Check sheet for the modelled part. Datum: model origin and axes. Units: mm. A direction names the side the tool comes from. Round coordinates to 2 decimals unless told otherwise and drop trailing zeros. Order: outer loops, then holes, each group sorted by start corner. A loop starts at its lowest first (then second) coordinate and runs counter-clockwise, first axis right, second up. Notation, with made-up numbers: M 69.5,9 L 84.5,9 A31 ccw 84.5,34 Z; hole C 56,-36.5 d7. An arc over 180 degrees is marked long. One line per item, written item: value. Start each with the question number.
(1) Access from +Z, -Z, +X, -X, +Y, -Y to the whole of each face (thin tool, end or side, straight path). Record for faces 4 (the face through (9, 1, 129)), 5 (the face through (90.51, 1.23, 121.35)).
(2) Cross-section at B-B, the plane x = 37.5. Enter the section's corners in (y, z), and give its area (3 significant figures).
(3) Thickness scan on L1, parallel to Z at x = 41, y = 1.75; L2, parallel to Z at x = 57, y = 1; L3, parallel to Z at x = 66, y = 1.3. Record the ranges inside material, lowest first.
(4) Cross-section at D-D, the plane x = 69. Enter the section's corners in (y, z), and give its area (3 significant figures).
(5) Cross-section at C-C, the plane z = 41. Enter the section's corners in (x, y), and give its area (3 significant figures).
(6) Cross-section at A-A, the plane z = 66. Enter the section's corners in (x, y), and give its area (3 significant figures).
(7) Release check for a two-part mould opening along Z. For faces 1 (the face through (15.65, 1.23, 121.51)), 2 (the face through (49, 0, 62)), 3 (the face through (97, 1, 8)) record: released by +Z, released by -Z, zero draft, split by the parting line, or undercut.
(8) Depth check by flat-ended pin: pin 1 Ø1 at (y, z) = (1, 75) entering from +X; pin 2 Ø0.8 at (x, y) = (72, 0.5) entering from -Z; pin 3 Ø1.1 at (x, z) = (-4.5, 112.5) entering from +Y; pin 4 Ø1.2 at (x, y) = (72.5, 1) entering from +Z. Enter the tip coordinate at first touch or a pass-through.
from build123d import *

# Parameters (mm, degrees)
SKETCH1_W               = 106
SKETCH1_H               = 137
BOSS_EXTRUDE1_DEPTH     = 2.5
CUT_EXTRUDE1_DEPTH      = 174.237553665
CUT_EXTRUDE1_DEPTH_BACK = 174.237553665
SKETCH5_W               = 8
SKETCH5_H               = 8
SKETCH5_R               = 0.9
SKETCH5_W_2             = 9
BOSS_EXTRUDE4_DEPTH     = 2.5
CUT_EXTRUDE4_DEPTH      = 181.818278943
CUT_EXTRUDE4_DEPTH_BACK = 181.818278943
SKETCH3_R               = 1.2
SKETCH3_W               = 6.263237977
SKETCH3_H               = 0.25
SKETCH3_W_2             = 4.268245837
CUT_EXTRUDE5_DEPTH      = 181.818278943
CUT_EXTRUDE5_DEPTH_BACK = 181.818278943
SKETCH7_W               = 30
SKETCH7_H               = 12


with BuildPart() as part:
    # Sketch1 → Boss-Extrude1 (new body)
    with BuildSketch(Plane(origin=(0, 0, 0), x_dir=(1, 0, 0), z_dir=(0, 1, 0))):
        with Locations((53, -68.5)):
            Rectangle(SKETCH1_W, SKETCH1_H)
    extrude(amount=BOSS_EXTRUDE1_DEPTH)

    # Sketch2 → Cut-Extrude1 (cut, two sides: drawn at the far end of the back side and taken through both)
    with BuildSketch(Plane(origin=(0, 2.5, 0), x_dir=(1, 0, 0), z_dir=(0, 1, 0)).offset(-CUT_EXTRUDE1_DEPTH_BACK)):
        Polygon((60.5, -83.5), (96, -83.5), (96, -115.857864376), (84.857864376, -127), (60.5, -127), align=None)
        Polygon((106, -120), (89, -137), (106, -137), align=None)
        Polygon((17, -137), (0, -120), (0, -137), align=None)
        Polygon((45.5, -127), (21.142135624, -127), (10, -115.857864376), (10, -83.5), (45.5, -83.5), align=None)
        Polygon((10, -53.5), (45.5, -53.5), (45.5, -8), (23.142135624, -8), (10, -21.142135624), align=None)
        Polygon((60.5, -53.5), (60.5, -8), (82.857864376, -8), (96, -21.142135624), (96, -53.5), align=None)
        Polygon((106, 0), (89, 0), (106, -17), align=None)
        Polygon((0, 0), (0, -17), (17, 0), align=None)
    extrude(amount=CUT_EXTRUDE1_DEPTH + CUT_EXTRUDE1_DEPTH_BACK, mode=Mode.SUBTRACT)

    # Sketch5 → Boss-Extrude4 (add)
    # profile 1 of 8: a face of its own
    with BuildSketch(Plane(origin=(0, 0, 0), x_dir=(1, 0, 0), z_dir=(0, 1, 0))):
        with Locations((22.5, -141)):
            Rectangle(SKETCH5_W, SKETCH5_H)
        with Locations(Location((22.5, -141, 0), (0, 0, 270))):
            Circle(SKETCH5_R, mode=Mode.SUBTRACT)
    # profile 2 of 8: a face of its own
    with BuildSketch(Plane(origin=(0, 0, 0), x_dir=(1, 0, 0), z_dir=(0, 1, 0))):
        with Locations((83.5, -141)):
            Rectangle(SKETCH5_W, SKETCH5_H)
        with Locations(Location((83.5, -141, 0), (0, 0, 270))):
            Circle(SKETCH5_R, mode=Mode.SUBTRACT)
    # profile 3 of 8: a face of its own
    with BuildSketch(Plane(origin=(0, 0, 0), x_dir=(1, 0, 0), z_dir=(0, 1, 0))):
        with Locations((83.5, 4)):
            Rectangle(SKETCH5_W, SKETCH5_H)
        with Locations(Location((83.5, 4, 0), (0, 0, 270))):
            Circle(SKETCH5_R, mode=Mode.SUBTRACT)
    # profile 4 of 8: a face of its own
    with BuildSketch(Plane(origin=(0, 0, 0), x_dir=(1, 0, 0), z_dir=(0, 1, 0))):
        with Locations((22.5, 4)):
            Rectangle(SKETCH5_W, SKETCH5_H)
        with Locations(Location((22.5, 4, 0), (0, 0, 270))):
            Circle(SKETCH5_R, mode=Mode.SUBTRACT)
    # profile 5 of 8: a face of its own
    with BuildSketch(Plane(origin=(0, 0, 0), x_dir=(1, 0, 0), z_dir=(0, 1, 0))):
        with Locations((-4.5, -112.5)):
            Rectangle(SKETCH5_W_2, SKETCH5_H)
        with Locations(Location((-4.5, -112.5, 0), (0, 0, 270))):
            Circle(SKETCH5_R, mode=Mode.SUBTRACT)
    # profile 6 of 8: a face of its own
    with BuildSketch(Plane(origin=(0, 0, 0), x_dir=(1, 0, 0), z_dir=(0, 1, 0))):
        with Locations((-4.5, -24.5)):
            Rectangle(SKETCH5_W_2, SKETCH5_H)
        with Locations(Location((-4.5, -24.5, 0), (0, 0, 270))):
            Circle(SKETCH5_R, mode=Mode.SUBTRACT)
    # profile 7 of 8: a face of its own
    with BuildSketch(Plane(origin=(0, 0, 0), x_dir=(1, 0, 0), z_dir=(0, 1, 0))):
        with BuildLine():
            Line((106, -113.4), (106, -116.5))
            Line((106, -116.5), (108, -116.5))
            Line((108, -116.5), (108, -108.5))
            Line((108, -108.5), (106, -108.5))
            Line((106, -108.5), (106, -111.6))
            ThreePointArc((106, -111.6), (106.9, -112.5), (106, -113.4))
        make_face()
    # profile 8 of 8: a face of its own
    with BuildSketch(Plane(origin=(0, 0, 0), x_dir=(1, 0, 0), z_dir=(0, 1, 0))):
        with BuildLine():
            Line((106, -25.4), (106, -28.5))
            Line((106, -28.5), (108, -28.5))
            Line((108, -28.5), (108, -20.5))
            Line((108, -20.5), (106, -20.5))
            Line((106, -20.5), (106, -23.6))
            ThreePointArc((106, -23.6), (106.9, -24.5), (106, -25.4))
        make_face()
    extrude(amount=BOSS_EXTRUDE4_DEPTH)

    # Sketch3 → Cut-Extrude4 (cut, two sides: drawn at the far end of the back side and taken through both)
    with BuildSketch(Plane(origin=(0, 2.5, 0), x_dir=(1, 0, 0), z_dir=(0, 1, 0)).offset(-CUT_EXTRUDE4_DEPTH_BACK)):
        with BuildLine():
            Line((56.27559049, -77.39), (56.27559049, -80.94))
            Line((56.27559049, -80.94), (98, -80.94))
            Line((98, -80.94), (98, -78.05675))
            ThreePointArc((98, -78.05675), (98.277140216, -77.040996997), (99.031754163, -76.30675))
            Line((99.031754163, -76.30675), (99.031754163, -76.05675))
            Line((99.031754163, -76.05675), (100, -76.05675))
            Line((100, -76.05675), (103.3, -76.05675))
            Line((103.3, -76.05675), (103.3, -60.94325))
            Line((103.3, -60.94325), (100, -60.94325))
            Line((100, -60.94325), (97.036762023, -60.94325))
            Line((97.036762023, -60.94325), (97.036762023, -60.69325))
            Line((97.036762023, -60.69325), (99.031754163, -60.69325))
            ThreePointArc((99.031754163, -60.69325), (98.277140216, -59.959003003), (98, -58.94325))
            Line((98, -58.94325), (98, -56.06))
            Line((98, -56.06), (56.27559049, -56.06))
            Line((56.27559049, -56.06), (56.27559049, -59.61))
            ThreePointArc((56.27559049, -59.61), (55.689804052, -61.024213562), (54.27559049, -61.61))
            Line((54.27559049, -61.61), (49.67559049, -61.61))
            Line((49.67559049, -61.61), (49.67559049, -75.39))
            Line((49.67559049, -75.39), (54.27559049, -75.39))
            ThreePointArc((54.27559049, -75.39), (55.689804052, -75.975786438), (56.27559049, -77.39))
        make_face()
        with Locations(Location((54.27559049, -59.61, 0), (0, 0, 270))):
            Circle(SKETCH3_R)
        with Locations(Location((54.27559049, -77.39, 0), (0, 0, 270))):
            Circle(SKETCH3_R)
        with Locations(Location((100, -78.05675, 0), (0, 0, 270))):
            Circle(SKETCH3_R)
        with Locations(Location((100, -58.94325, 0), (0, 0, 270))):
            Circle(SKETCH3_R)
        with Locations((100.168381012, -60.81825)):
            Rectangle(SKETCH3_W, SKETCH3_H)
        with Locations((101.165877082, -76.18175)):
            Rectangle(SKETCH3_W_2, SKETCH3_H)
    extrude(amount=CUT_EXTRUDE4_DEPTH + CUT_EXTRUDE4_DEPTH_BACK, mode=Mode.SUBTRACT)

    # Sketch7 → Cut-Extrude5 (cut, two sides: drawn at the far end of the back side and taken through both)
    with BuildSketch(Plane(origin=(0, 2.5, 0), x_dir=(1, 0, 0), z_dir=(0, 1, 0)).offset(-CUT_EXTRUDE5_DEPTH_BACK)):
        with Locations((34.67559049, -68.5)):
            Rectangle(SKETCH7_W, SKETCH7_H)
    extrude(amount=CUT_EXTRUDE5_DEPTH + CUT_EXTRUDE5_DEPTH_BACK, mode=Mode.SUBTRACT)


solid = part.part
Values found:
1. face 4: +Z, -X, +Y, -Y
1. face 5: +Y, -Y
2. outline: M 0,0 L 2.5,0 L 2.5,8 L 0,8 Z; M 0,53.5 L 2.5,53.5 L 2.5,62.5 L 0,62.5 Z; M 0,74.5 L 2.5,74.5 L 2.5,83.5 L 0,83.5 Z; M 0,127 L 2.5,127 L 2.5,137 L 0,137 Z
2. area: 90.0 mm^2
3. L1: 0 to 8, 53.5 to 62.5, 74.5 to 83.5, 127 to 137
3. L2: 0 to 56.06, 80.94 to 137
3. L3: 0 to 8, 53.5 to 56.06, 80.94 to 83.5, 127 to 137
4. outline: M 0,0 L 2.5,0 L 2.5,8 L 0,8 Z; M 0,53.5 L 2.5,53.5 L 2.5,56.06 L 0,56.06 Z; M 0,80.94 L 2.5,80.94 L 2.5,83.5 L 0,83.5 Z; M 0,127 L 2.5,127 L 2.5,137 L 0,137 Z
4. area: 57.8 mm^2
5. outline: M 0,0 L 10,0 L 10,2.5 L 0,2.5 Z; M 45.5,0 L 60.5,0 L 60.5,2.5 L 45.5,2.5 Z; M 96,0 L 106,0 L 106,2.5 L 96,2.5 Z
5. area: 87.5 mm^2
6. outline: M 0,0 L 19.68,0 L 19.68,2.5 L 0,2.5 Z; M 103.3,0 L 106,0 L 106,2.5 L 103.3,2.5 Z
6. area: 55.9 mm^2
7. face 1: undercut
7. face 2: zero draft
7. face 3: released by -Z
8. pin 1: x = 106
8. pin 2: z = 0
8. pin 3: through
8. pin 4: z = 137
